Study the drawing (mm; zero at the part's minimum x, y, z) and answer. A direction names the side the tool comes from. Coordinates: 2 decimals unless noted, no trailing zeros. Loops run counter-clockwise (first coordinate to the right, second up) from the corner with the lowest first, then second, coordinate; pieces in that order, holes last. Notation, with made-up numbers: (54.25, 2) -> (88.25, 2) arc R23 ccw to (88.25, 33) -> close; hole circle Ø9 at (-19.5, 58.25). An arc over 180 degrees is marked (long way). Answer as CSV lines item,"result".
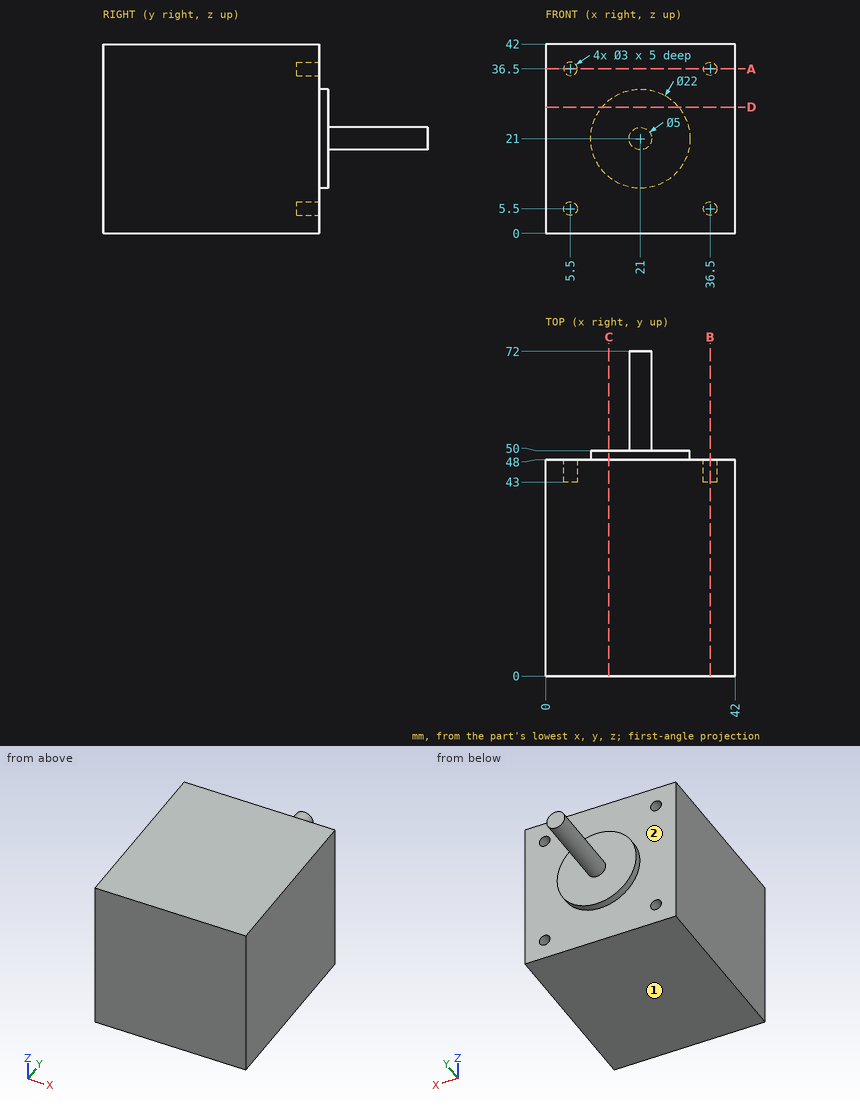
Q1. A cutting plane is placed at D-D, the plane z = 28. Write down the section's boundary in (x, y), and give its area (3 significant figures).
Results:
outline,"(0, 0) -> (42, 0) -> (42, 48) -> (29.49, 48) -> (29.49, 50) -> (12.51, 50) -> (12.51, 48) -> (0, 48) -> close"
area,"2,050 mm²"
Q2. A cutting plane is placed at B-B, the plane x = 36.5. Write down the section's boundary in (y, z).
Results:
outline,"(0, 0) -> (48, 0) -> (48, 4) -> (43, 4) -> (43, 7) -> (48, 7) -> (48, 35) -> (43, 35) -> (43, 38) -> (48, 38) -> (48, 42) -> (0, 42) -> close"
Q3. Given pin 1 Ø2.5 at (x, z) = (37, 5.5) entering from +Y; pin 2 Ø1.8 at (x, z) = (5.5, 5.5) entering from +Y; pin 3 Ø10 at (y, z) = (64.5, 16.5) entering from +X; pin 4 Ø10 at (x, y) = (13, 63) entering from -Z, each flat-ended and moving along its own axis, determine where each tip first touches the part or whether it passes through.
Results:
pin 1,"stops at y = 48"
pin 2,"stops at y = 43"
pin 3,"stops at x = 23.5"
pin 4,"passes through"
Q4. A cutting plane is placed at A-A, the plane z = 36.5. Write down the section's boundary in (x, y), and give its area (3 significant figures).
Results:
outline,"(0, 0) -> (42, 0) -> (42, 48) -> (38, 48) -> (38, 43) -> (35, 43) -> (35, 48) -> (7, 48) -> (7, 43) -> (4, 43) -> (4, 48) -> (0, 48) -> close"
area,"1,990 mm²"
Q5. Find the intervals of material crossed by probe 1 along Z at (x, y) = (5.5, 45.5); probe 2 along X at (y, z) = (44, 36), in increasing order. Write a range as [from, to].
Results:
probe 1,"z = [0, 4], [7, 35], [38, 42]"
probe 2,"x = [0, 4.09], [6.91, 35.09], [37.91, 42]"
Q6. For the marked faces 1 and 2, determine the directions among +Z, -Z, +X, -X, +Y, -Y from which every point of the face is accessible in a straight line to the end or side of a thin tool.
Results:
face 1,"-Z, +X, -X, +Y, -Y"
face 2,"+Y"
Q7. A cutting plane is placed at C-C, the plane x = 14. Write down the section's boundary in (y, z), and give its area (3 significant figures).
Results:
outline,"(0, 0) -> (48, 0) -> (48, 12.51) -> (50, 12.51) -> (50, 29.49) -> (48, 29.49) -> (48, 42) -> (0, 42) -> close"
area,"2,050 mm²"
